Drawing for the job (mm, zero at the part's lowest x, y, z). A direction names the side the tool comes from. Round coordinates to 2 decimals unless told otherwise and drop trailing zeros. Write each loop counter-clockwise with the first axis right and the second up, starting at its lowest first coordinate (ties: lowest second). Pieces come first, ordered by that corner, then holes. Notation, with made-up numbers: (55.25, 4.5) - (86.25, 4.5) arc R24 ccw to (86.25, 19.5) - close; hole circle Ø1 at (36, 82.5). An arc over 180 degrees is marked (long way). Answer in a Markdown table with one row per item.
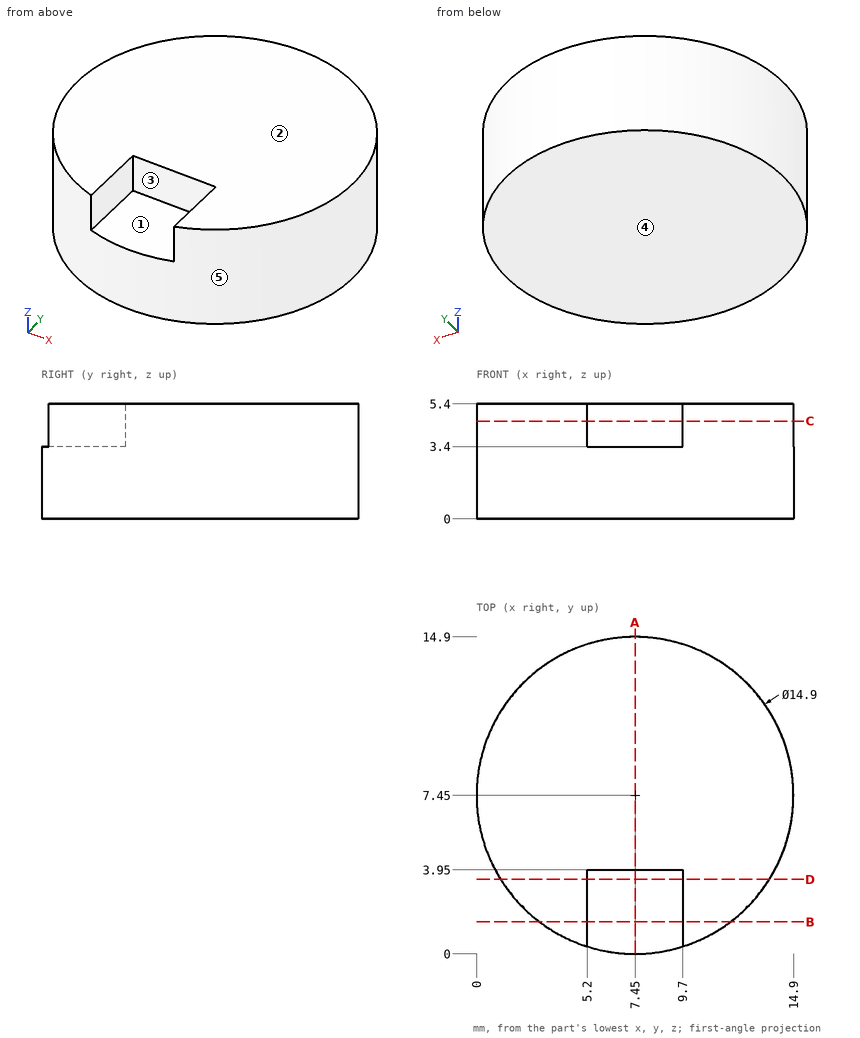
Q1. Flat gauge pins, fed straight in: pin 1 (2 mm diameter, centred on x = 8, z = 4.5, fed in from -Y); pin 2 (1.5 mm diameter, centred on x = 4.5, y = 6, fed in from -Z); pin 3 (1 mm diameter, centred on y = 2, z = 4, fed in from -X); pin 4 (1 mm diameter, centred on y = 3.5, z = 1.5, fed in from -X). Where does each tip first touch, or does it go through?
Computed:
| item | result |
|---|---|
| pin 1 | stops at y = 3.95 |
| pin 2 | stops at z = 0 |
| pin 3 | stops at x = 1.88 |
| pin 4 | stops at x = 0.85 |
Q2. Pull direction X, two halves, no side cores. Call the marked faces 3, 4 and 5: released by +X, released by -X, zero draft, split by the parting line, or undercut.
Computed:
| item | result |
|---|---|
| face 3 | undercut |
| face 4 | zero draft |
| face 5 | split by the parting line |
Q3. 3-axis set-ups, long thin cutter, end or side, ignore diameter. For the marked faces 1 and 2: which of +Z, -Z, +X, -X, +Y, -Y reach the whole face in a straight line?
Computed:
| item | result |
|---|---|
| face 1 | +Z, -Y |
| face 2 | +Z, +X, -X, +Y, -Y |
Q4. Saw through at A-A on x = 7.45. List the corners of the cut face in (y, z).
Computed:
| item | result |
|---|---|
| outline | (0, 0) - (14.9, 0) - (14.9, 5.4) - (3.95, 5.4) - (3.95, 3.4) - (0, 3.4) - close |
Q5. Saw through at D-D on y = 3.5. List the corners of the cut face in (x, z), then the cut area to 3 significant figures.
Computed:
| item | result |
|---|---|
| outline | (1.13, 0) - (13.77, 0) - (13.77, 5.4) - (9.7, 5.4) - (9.7, 3.4) - (5.2, 3.4) - (5.2, 5.4) - (1.13, 5.4) - close |
| area | 59.2 mm2 |
Q6. Saw through at C-C on z = 4.6. List the corners of the cut face in (x, y).
Computed:
| item | result |
|---|---|
| outline | (5.2, 0.35) - (5.2, 3.95) - (9.7, 3.95) - (9.7, 0.35) arc R7.45 ccw (long way) to start |
Q7. Saw through at B-B on y = 1.5. List the corners of the cut face in (x, z), then the cut area to 3 significant figures.
Computed:
| item | result |
|---|---|
| outline | (2.97, 0) - (11.93, 0) - (11.93, 5.4) - (9.7, 5.4) - (9.7, 3.4) - (5.2, 3.4) - (5.2, 5.4) - (2.97, 5.4) - close |
| area | 39.4 mm2 |
Q8. Drill centre lines: line 1 (Z direction, x = 8.75, y = 3.75); line 2 (X direction, y = 2.25, z = 3.95); line 3 (X direction, y = 12.75, z = 3.2). Where is each one in solid material? Low to high.
Computed:
| item | result |
|---|---|
| line 1 | z = 0 to 3.4 |
| line 2 | x = 2.11 to 5.2, 9.7 to 12.79 |
| line 3 | x = 2.21 to 12.69 |
